Input: dimensioned drawing with shaded views. Units: mm. Origin: part minimum x, y, z. A direction names the side the tool comes from. Round coordinates to 2 decimals unless told otherwise and drop trailing zeros. Loops run counter-clockwise (first coordinate to the right, second up) from the corner with the lowest first, then second, coordinate; pieces in that order, holes last. Notation, with made-up numbers: M 71,9.25 L 87,9.25 A23 ccw 87,35.25 Z; hole C 88.5,-18.75 d7. An arc over 180 degrees is marked long. Put each result on its own line as item: value. Start each with the question number.
1) Line query: probe 1 along X at (y, z) = (204, 15.5); probe 2 along X at (y, z) = (153.5, 115); probe 3 along Y at (x, z) = (756, 135). Output: solid intervals per line, ascending.
2) Section A-A on z = 100. Output: boundary loops of the cut face in (x, y), plus the area to 3 significant figures.
3) Pin query (flat end, axial travel): pin 1 (4 mm diameter, centred on y = 36, z = 44.5, fed in from +X); pin 2 (20 mm diameter, centred on x = 717.5, z = 119.5, fed in from -Y); pin 3 (1.5 mm diameter, centred on y = 54.5, z = 125, fed in from +X). Return the tip coordinate at first contact, or that it passes through.
4) Section C-C on y = 74. Output: boundary loops of the cut face in (x, z), plus the area to 3 significant figures.
5) Reachability of the marked faces 1, 2 and 3 from +Z, -Z, +X, -X, +Y, -Y: full face, straight path, thin tool, end or side. Return the list, or none.
6) Section B-B on y = 123. Output: boundary loops of the cut face in (x, z).
7) Section D-D on z = 14.5. Output: boundary loops of the cut face in (x, y), plus the area to 3 significant figures.
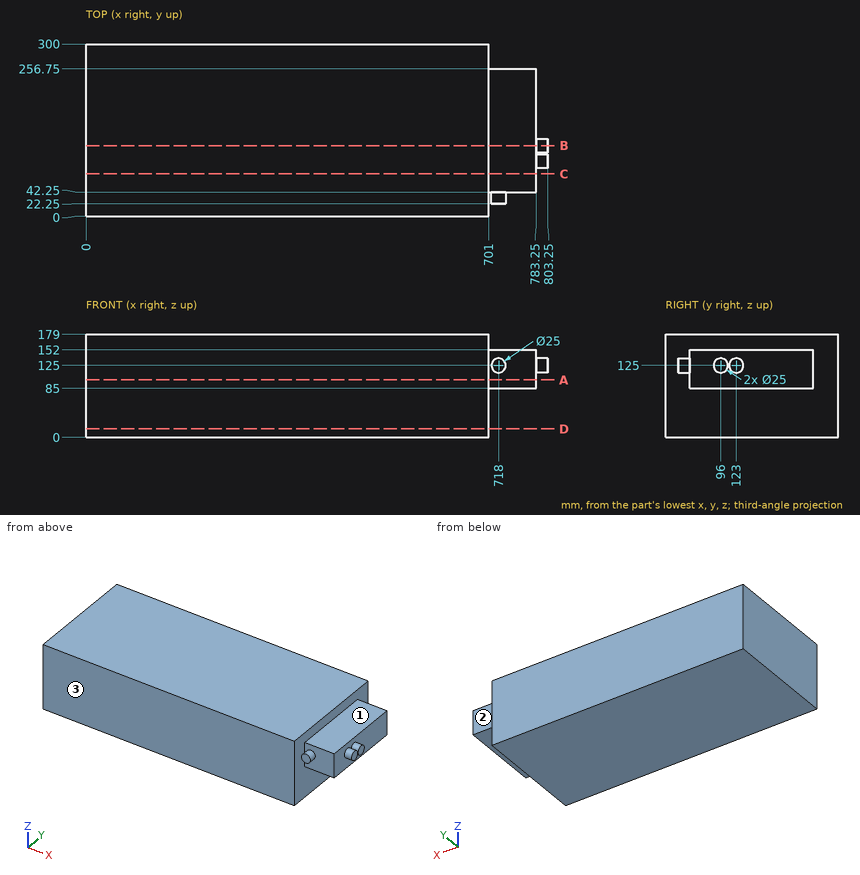
Geometry results:
1. probe 1: x = 0 to 701
1. probe 2: x = 0 to 783.25
1. probe 3: y = 42.25 to 256.75
2. outline: M 0,0 L 701,0 L 701,42.25 L 783.25,42.25 L 783.25,256.75 L 701,256.75 L 701,300 L 0,300 Z
2. area: 228,000 mm²
3. pin 1: stops at x = 701
3. pin 2: stops at y = 22.25
3. pin 3: stops at x = 783.25
4. outline: M 0,0 L 701,0 L 701,85 L 783.25,85 L 783.25,152 L 701,152 L 701,179 L 0,179 Z
4. area: 131,000 mm²
5. face 1: +Z, +X, +Y, -Y
5. face 2: +Z, -Z, +X, +Y
5. face 3: +Z, -Z, +X, -X, -Y
6. outline: M 0,0 L 701,0 L 701,85 L 783.25,85 L 783.25,112.5 L 803.25,112.5 L 803.25,137.5 L 783.25,137.5 L 783.25,152 L 701,152 L 701,179 L 0,179 Z
7. outline: M 0,0 L 701,0 L 701,300 L 0,300 Z
7. area: 210,000 mm²
